Geometry check sheet. Reference: the model listing, model coordinates, mm. A direction names the side the tool comes from. Coordinates: 2 decimals unless noted, no trailing zeros. Write each loop counter-clockwise with the first axis right and the second up, starting at its lowest first coordinate (ties: lowest second). Pieces come first, ordered by that corner, then holes. Notation, with made-up numbers: (16.5, -3.75) -> (47.5, -3.75) arc R22 cw to (47.5, 10.25) -> close; hole circle Ø10 at (70.5, 73.5). An arc over 180 degrees is marked (long way). Answer in a Markdown table with one row per item. Add a question column.
1. Cross-section at C-C on x = 87. Record the cut outline in (y, z), and give its area (3 significant figures).
2. Scan lines: L1, parallel to Y at x = 30.5, z = 38; L2, parallel to X at y = 4.5, z = 35; L3, parallel to X at y = -86, z = 37. Record each from-to range of solid material in increasing order. Write a range as from..to.
3. Cross-section at B-B on z = 22.5. Record the cut outline in (x, y), and give its area (3 significant figures).
4. Set-up check for faces 1 (the flat face through (20, -1, 25)), 2 (the flat face through (-1, -125, 25)): record each of +Z, -Z, +X, -X, +Y, -Y from which the full face is reachable in a straight line by a thin tool's end or side.
5. Cross-section at D-D on y = -85. Record the cut outline in (x, z).
6. Mould release check, pull along X, two halves, no side actions. Record for faces 3 (the flat face through (10, -1, 25)), 4 (the flat face through (14, -32, 50)), 5 (the flat face through (-100, -26, 25)), 6 (the flat face through (100, -26, 25)): pulls with the +X half, pulls with the -X half, needs draft (parallel to the pull), parting line crosses it, or undercut.
7. Cross-section at A-A on y = -47.5. Record the cut outline in (x, z).
```python
from build123d import *

# Parameters (mm, degrees)
SKETCH1_W           = 10
SKETCH1_H           = 40
SKETCH1_H_2         = 10
SKETCH1_W_2         = 180
SKETCH1_W_3         = 200
SKETCH1_H_3         = 150
SKETCH1_W_4         = 100
SKETCH1_H_4         = 130
SKETCH1_W_5         = 70
BOSS_EXTRUDE1_DEPTH = 50


with BuildPart() as part:
    # Sketch1 → Boss-Extrude1 (new body)
    # profile 1 of 6: a face of its own
    with BuildSketch(Plane.XY):
        with Locations((-95, -95)):
            Rectangle(SKETCH1_W, SKETCH1_H)
    # profile 2 of 6: a face of its own
    with BuildSketch(Plane.XY):
        with Locations((-95, -120)):
            Rectangle(SKETCH1_W, SKETCH1_H_2)
    # profile 3 of 6: a face of its own
    with BuildSketch(Plane.XY):
        with Locations((0, -120)):
            Rectangle(SKETCH1_W_2, SKETCH1_H_2)
    # profile 4 of 6: a face of its own
    with BuildSketch(Plane.XY):
        with Locations((95, -120)):
            Rectangle(SKETCH1_W, SKETCH1_H_2)
    # profile 5 of 6: a face of its own
    with BuildSketch(Plane.XY):
        with Locations((95, -95)):
            Rectangle(SKETCH1_W, SKETCH1_H)
    # profile 6 of 6: a face of its own
    with BuildSketch(Plane.XY):
        Rectangle(SKETCH1_W_3, SKETCH1_H_3)
        with Locations((-40, 0)):
            Rectangle(SKETCH1_W_4, SKETCH1_H_4, mode=Mode.SUBTRACT)
        with Locations((55, 0)):
            Rectangle(SKETCH1_W_5, SKETCH1_H_4, mode=Mode.SUBTRACT)
    extrude(amount=BOSS_EXTRUDE1_DEPTH)


solid = part.part
```
Results found:
| question | item | result |
|---|---|---|
| 1 | outline | (-125, 0) -> (-115, 0) -> (-115, 50) -> (-125, 50) -> close; (-75, 0) -> (-65, 0) -> (-65, 50) -> (-75, 50) -> close; (65, 0) -> (75, 0) -> (75, 50) -> (65, 50) -> close |
| 1 | area | 1,500 mm^2 |
| 2 | L1 | y = -125..-115, -75..-65, 65..75 |
| 2 | L2 | x = -100..-90, 10..20, 90..100 |
| 2 | L3 | x = -100..-90, 90..100 |
| 3 | outline | (-100, -125) -> (100, -125) -> (100, 75) -> (-100, 75) -> close; hole (-90, -115) -> (90, -115) -> (90, -75) -> (-90, -75) -> close; hole (-90, -65) -> (10, -65) -> (10, 65) -> (-90, 65) -> close; hole (20, -65) -> (90, -65) -> (90, 65) -> (20, 65) -> close |
| 3 | area | 10,700 mm^2 |
| 4 | face 1 | +Z, -Z |
| 4 | face 2 | +Z, -Z, +X, -X, -Y |
| 5 | outline | (-100, 0) -> (-90, 0) -> (-90, 50) -> (-100, 50) -> close; (90, 0) -> (100, 0) -> (100, 50) -> (90, 50) -> close |
| 6 | face 3 | undercut |
| 6 | face 4 | needs draft |
| 6 | face 5 | pulls with the -X half |
| 6 | face 6 | pulls with the +X half |
| 7 | outline | (-100, 0) -> (-90, 0) -> (-90, 50) -> (-100, 50) -> close; (10, 0) -> (20, 0) -> (20, 50) -> (10, 50) -> close; (90, 0) -> (100, 0) -> (100, 50) -> (90, 50) -> close |
